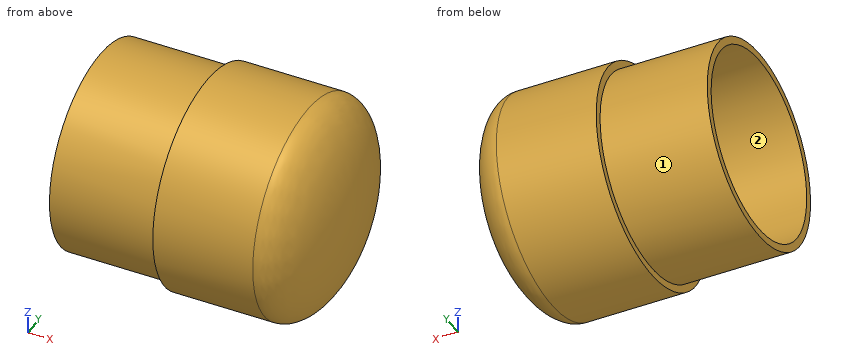
from build123d import *


with BuildPart() as part:
    # Sketch1 → Revolve1 (revolve)
    with BuildSketch(Plane.XY, mode=Mode.PRIVATE) as revolve1_sk:
        with BuildLine():
            Line((-138.90625, -109.5375), (-21.43125, -109.5375))
            Line((-21.43125, -109.5375), (-21.43125, -117.7163))
            Line((-21.43125, -117.7163), (88.10625, -117.7163))
            add(Edge.make_bspline(
                [(88.10625, -117.7163), (138.90625, -117.7163), (138.90625, 0)],
                knots=[3.141592654, 3.141592654, 3.141592654, 4.71238898, 4.71238898, 4.71238898], degree=2, weights=[1, 0.707106781, 1]))
            Line((138.90625, 0), (130.72745, 0))
            add(Edge.make_bspline(
                [(88.10625, -101.3587), (130.72745, -101.3587), (130.72745, 0)],
                knots=[0, 0, 0, 1.570796327, 1.570796327, 1.570796327], degree=2, weights=[1, 0.707106781, 1]))
            Line((88.10625, -101.3587), (-138.90625, -101.3587))
            Line((-138.90625, -101.3587), (-138.90625, -109.5375))
        make_face()
    revolve(revolve1_sk.sketch.rotate(Axis((-138.90625, 0, 0), (1, 0, 0)), 270), axis=Axis((-138.90625, 0, 0), (1, 0, 0)))


solid = part.part
For this review, take the finished solid that the model builds, in its own axes (mm). Face numbers are marked on the shaded views. Coordinates: 2 decimals unless noted, no trailing zeros. Order: outer loops, then holes, each group sorted by start corner. A loop starts at its lowest first (then second) coordinate and runs counter-clockwise, first axis right, second up. Notation, with made-up numbers: (84.5, 64) -> (139.5, 64) arc R26 cw to (139.5, 100) -> close; hole circle Ø11 at (68, 15). An arc over 180 degrees is marked (long way). Return JSON: item names as keys, results as strings.
1. For pin 1 Ø10 at (x, y) = (-47.5, -66.5) entering from -Z; pin 2 Ø5 at (x, y) = (80.5, -75.5) entering from -Z; pin 3 Ø1.5 at (x, z) = (-68, -73) entering from -Y, all flat-tipped, find the tip position at first contact; note any pin that passes through.
Answer block:
{"pin 1": "z = -90.64", "pin 2": "z = -92.35", "pin 3": "y = -82.33"}
2. We need section A-A on x = -28.5. Write out the cut boundary in (y, z) (1 decimal).
Answer block:
{"outline": "circle Ø219.1 at (0, 0); hole circle Ø202.7 at (0, 0)"}
3. The part is to be moulded in two halves that separate along Z. For the marked faces 1 and 2, say which applies: +Z half, -Z half, draft (parallel to the pull), parting line (faces both ways), or undercut.
Answer block:
{"face 1": "parting line", "face 2": "undercut"}
4. For line 1 (Y direction, x = -39.5, z = 0); line 2 (Y direction, x = -19, z = 0); line 3 (Z direction, x = 1, y = -59), list the stretches that pass through material, from the lowest coordinate up. Write a range as from..to.
Answer block:
{"line 1": "-109.54..-101.36, 101.36..109.54", "line 2": "-117.72..-101.36, 101.36..117.72", "line 3": "-101.86..-82.42, 82.42..101.86"}
